```python
from build123d import *

# Parameters (mm, degrees)
BOSS_EXTRUDE1_DEPTH = 20
SHELL2_T            = -4


with BuildPart() as part:
    # Sketch2 → Boss-Extrude1 (new body)
    with BuildSketch(Plane(origin=(-1e-09, -0.00010259, -0.052603991), x_dir=(1, 0, -1.2e-08), z_dir=(1.2e-08, 0.001950226, 0.999998098))):
        Polygon((-75.063999083, -32.893592991), (-67.504997012, -32.893592991), (4.936001691, -32.893592991), (4.936001691, 32.106283405), (-2.495998153, 32.10628351), (-62.495998239, 32.106284359), (-75.063999083, 32.106284359), align=None)
    extrude(amount=BOSS_EXTRUDE1_DEPTH)

    # Shell2
    shell2_openings = [part.faces().sort_by_distance(p)[0] for p in [
        (-40.55039837, 6.145223556, 19.93544972),
    ]]
    offset(amount=SHELL2_T, openings=shell2_openings, kind=Kind.INTERSECTION)


solid = part.part
```
Model file for the job. Use its own axes, mm. Give positions to 0.01 mm unless a question says otherwise; leave off trailing zeros. Order: outer loops, then holes, each group sorted by start corner. A loop starts at its lowest first (then second) coordinate and runs counter-clockwise, first axis right, second up.
1) Saw through at C-C, the plane y = -2. Write the cut outline in (x, z), then the cut area to 3 significant figures.
2) Wall check: probe 1 along Y at (x, z) = (-12, 13.5); probe 2 along X at (y, z) = (19.5, 11.25); probe 3 along Y at (x, z) = (-3.5, 2.25). Give the ranges that are in metal, low to high.
3) Saw through at A-A, the plane x = -18. Write the cut outline in (y, z), then the cut area to 3 significant figures.
4) Pin check, flat tips, straight feed: pin 1 (2 mm diameter, centred on x = -3.5, z = 15, fed in from +Y); pin 2 (12 mm diameter, centred on x = -55.5, y = -10.5, fed in from +Z); pin 3 (1 mm diameter, centred on x = -8.5, y = 2, fed in from -Z). Stop position of each tip, or through.
5) Mould opens along Y. For faces 1 (the flat face through (4.936, -1, 10)), 2 (the flat face through (0.936, -1, 12)), 3 (the flat face through (-71.064, 0, 12)) say: +Y half, -Y half, draft (parallel to the pull), parting line (faces both ways), or undercut.
6) Saw through at B-B, the plane z = 17. Write the cut outline in (x, y), then the cut area to 3 significant figures.
Computed:
1. outline: (-75.06, -0.05) - (4.94, -0.05) - (4.94, 19.95) - (0.94, 19.95) - (0.94, 3.95) - (-71.06, 3.95) - (-71.06, 19.95) - (-75.06, 19.95) - close
1. area: 448 mm2
2. probe 1: y = -32.87 to -28.87, 28.13 to 32.13
2. probe 2: x = -75.06 to -71.06, 0.94 to 4.94
2. probe 3: y = -32.89 to 32.11
3. outline: (-32.89, 0.01) - (32.11, -0.12) - (32.15, 19.88) - (28.15, 19.89) - (28.11, 3.89) - (-28.89, 4) - (-28.85, 20) - (-32.85, 20.01) - close
3. area: 388 mm2
4. pin 1: stops at y = 32.14
4. pin 2: stops at z = 3.98
4. pin 3: stops at z = -0.06
5. face 1: draft
5. face 2: undercut
5. face 3: undercut
6. outline: (-75.06, -32.86) - (4.94, -32.86) - (4.94, 32.14) - (-75.06, 32.14) - close; hole (-71.06, -28.86) - (0.94, -28.86) - (0.94, 28.14) - (-71.06, 28.14) - close
6. area: 1,100 mm2
